from build123d import *

# Parameters (mm, degrees)
BOSS_EXTRUDE1_DEPTH     = 212
BOSS_EXTRUDE2_DEPTH     = 10
BOSS_EXTRUDE3_DEPTH     = 10
SKETCH4_R               = 3
CUT_EXTRUDE1_DEPTH      = 91
SKETCH6_R               = 7.5
CUT_EXTRUDE2_DEPTH      = 81
SKETCH7_R               = 1.5
SKETCH7_R_2             = 12.5
SKETCH7_W               = 10
SKETCH7_H               = 120
SKETCH7_W_2             = 60
SKETCH7_H_2             = 15
CUT_EXTRUDE3_DEPTH      = 12.5
CUT_EXTRUDE4_REACH      = 112.512
SKETCH8_R               = 12.5
SKETCH9_R               = 3
CUT_EXTRUDE5_DEPTH      = 26
CUT_EXTRUDE5_DEPTH_BACK = 66
SKETCH10_W              = 40
SKETCH10_H              = 6.35
CUT_EXTRUDE6_DEPTH      = 1
CUT_EXTRUDE6_DEPTH_BACK = 213
FILLET1_R               = 10


with BuildPart() as part:
    # Sketch1 → Boss-Extrude1 (new body)
    with BuildSketch(Plane.XY):
        Polygon((0, 0), (-20, 0), (-20, 20), (-242.984559153, 20), (-242.984559153, 25), (-260, 25), (-260, 30), (-49.158083864, 30), (-122.301669645, 77.5), (-242.984559153, 85), (-260, 85), (-260, 90), (-242.984559153, 90), (-110.511971445, 81.767313396), (0, 10), align=None)
    extrude(amount=BOSS_EXTRUDE1_DEPTH)

    # Sketch2 → Boss-Extrude2 (add)
    with BuildSketch(Plane(origin=(0, 0, 0), x_dir=(-1, 0, 0), z_dir=(0, 0, -1))):
        Polygon((0, 0), (260, 0), (260, 90), (110.511971445, 81.767313396), (0, 10), align=None)
    extrude(amount=-BOSS_EXTRUDE2_DEPTH)

    # Sketch3 → Boss-Extrude3 (add)
    with BuildSketch(Plane.XY.offset(212)):
        Polygon((-110.511971445, 81.767313396), (0, 10), (0, 0), (-260, 0), (-260, 90), align=None)
    extrude(amount=-BOSS_EXTRUDE3_DEPTH)

    # Sketch4 → Cut-Extrude1 (cut, through all)
    with BuildSketch(Plane.XZ):
        with Locations((-10, 187)):
            Circle(SKETCH4_R)
        with Locations((-10, 25)):
            Circle(SKETCH4_R)
    extrude(amount=-CUT_EXTRUDE1_DEPTH, mode=Mode.SUBTRACT)

    # Sketch6 → Cut-Extrude2 (cut, through all)
    with BuildSketch(Plane(origin=(0, 10, 0), x_dir=(-1, 0, 0), z_dir=(0, -1, 0))):
        with Locations((10, -25)):
            Circle(SKETCH6_R)
        with Locations((10, -187)):
            Circle(SKETCH6_R)
    extrude(amount=-CUT_EXTRUDE2_DEPTH, mode=Mode.SUBTRACT)

    # Sketch7 → Cut-Extrude3 (cut)
    with BuildSketch(Plane.XZ.offset(-20)):
        with Locations((-161.484559153, 161)):
            Circle(SKETCH7_R)
        with Locations((-225.684559153, 161)):
            Circle(SKETCH7_R)
        with Locations((-161.484559153, 51)):
            Circle(SKETCH7_R)
        with Locations((-225.684559153, 51)):
            Circle(SKETCH7_R)
        with Locations((-67.984559153, 136)):
            Circle(SKETCH7_R_2)
        with Locations((-92.099111311, 106)):
            Rectangle(SKETCH7_W, SKETCH7_H)
        with Locations((-70, 22.5)):
            Rectangle(SKETCH7_W_2, SKETCH7_H_2)
    extrude(amount=-CUT_EXTRUDE3_DEPTH, mode=Mode.SUBTRACT)

    # Sketch8 → Cut-Extrude4 (cut, up to next)
    with BuildSketch(Plane.ZY.offset(110.511971445), mode=Mode.PRIVATE) as cut_extrude4_sk1:
        with Locations((54, 57.25)):
            Circle(SKETCH8_R)
    cut_extrude4_tool1 = extrude(cut_extrude4_sk1.sketch, amount=-CUT_EXTRUDE4_REACH, mode=Mode.PRIVATE) & part.part
    add(cut_extrude4_tool1.solids().sort_by_distance((-110.511971, 57.25, 54))[0], mode=Mode.SUBTRACT)

    # Sketch9 → Cut-Extrude5 (cut, two sides)
    with BuildSketch(Plane.XZ.offset(-25)) as cut_extrude5_sk:
        with Locations((-251.5, 182)):
            Circle(SKETCH9_R)
        with Locations((-251.5, 30)):
            Circle(SKETCH9_R)
    extrude(amount=CUT_EXTRUDE5_DEPTH, mode=Mode.SUBTRACT)
    extrude(cut_extrude5_sk.sketch, amount=-CUT_EXTRUDE5_DEPTH_BACK, mode=Mode.SUBTRACT)

    # Sketch10 → Cut-Extrude6 (cut, two sides)
    with BuildSketch(Plane.XY.offset(212)) as cut_extrude6_sk:
        with Locations((-107.5, 3.175)):
            Rectangle(SKETCH10_W, SKETCH10_H)
    extrude(amount=CUT_EXTRUDE6_DEPTH, mode=Mode.SUBTRACT)
    extrude(cut_extrude6_sk.sketch, amount=-CUT_EXTRUDE6_DEPTH_BACK, mode=Mode.SUBTRACT)

    # Fillet1
    fillet1_edges = [part.edges().sort_by_distance(p)[0] for p in [
        (-110.511971445, 81.767313396, 106),
    ]]
    fillet(fillet1_edges, radius=FILLET1_R)


solid = part.part
Design review of the part built by this model. Coordinates are the model's own, in mm. A direction names the side the tool comes from. Round coordinates to 2 decimals unless told otherwise and drop trailing zeros. Loops run counter-clockwise (first coordinate to the right, second up) from the corner with the lowest first, then second, coordinate; pieces in that order, holes last. Notation, with made-up numbers: (38, 20.5) -> (68, 20.5) arc R27 ccw to (68, 44.5) -> close; hole circle Ø2 at (11, 50). An arc over 180 degrees is marked (long way). Use one line per item in the form item = value. Start each with the question number.
Q1. For pin 1 Ø6 at (x, z) = (-161, 100.5) entering from +Y; pin 2 Ø1.5 at (x, z) = (-110.5, 59.5) entering from +Y; pin 3 Ø2 at (y, z) = (74.5, 108.5) entering from +X; pin 4 Ø5.5 at (x, z) = (-251.5, 182) entering from -Y, all flat-tipped, find the tip position at first contact; note any pin that passes through.
Q2. We need section C-C on y = 65.5. Give the boundary of the cut face in (x, z), then the cut area to 3 significant figures.
Q3. We need section B-B on z = 117. Give the boundary of the cut face in (x, y), then the cut area to 3 significant figures.
Q4. We need section A-A on x = -251.5. Give the boundary of the cut face in (y, z), then the cut area to 3 significant figures.
Q5. Draft analysis for pull direction X (two halves, no side actions). For faces 6 (the face through (-157, 36, 212)), 7 (the face through (-108, 6.35, 5)), 8 (the face through (-20, 10, 105)), state which applies: +X half, -X half, draft (parallel to the pull), parting line (faces both ways), or undercut.
Q6. Wall thickness on line 1 along Z through (x, y) = (-251, 28); line 2 along Z through (x, y) = (-207, 10); line 3 along Y through (x, z) = (-190.5, 166.5): over which ranges is each line inside the solid? List them lowest first. Write a range as [from, to].
Q7. Machinability: for faces 1 (the face through (-17.154, 14.34, 22.747)), 2 (the face through (-127.5, 3, 207)), 3 (the face through (-87.099, 25, 105)), 4 (the face through (0, 5, 105)), 5 (the face through (-47, 32.5, 23)), which of the approach directions +Z, -Z, +X, -X, +Y, -Y give a long, thin tool a straight path to every point of the face, cutting with its end or side? Answer none if there is none.
Q8. We need section D-D on x = -10. Give the boundary of the cut face in (y, z).
Calculated:
q1.pin_1 = 85.09
q1.pin_2 = 81.63
q1.pin_3 = -97.78
q1.pin_4 = through
q2.outline = (-260, 0) -> (-85.46, 0) -> (-85.46, 44.61) -> (-103.82, 44.61) -> (-103.82, 10) -> (-260, 10) -> close; (-260, 202) -> (-103.82, 202) -> (-103.82, 63.39) -> (-85.46, 63.39) -> (-85.46, 212) -> (-260, 212) -> close
q2.area = 6,670 mm²
q3.outline = (-260, 25) -> (-242.98, 25) -> (-242.98, 20) -> (-97.1, 20) -> (-97.1, 30) -> (-260, 30) -> close; (-260, 85) -> (-242.98, 85) -> (-122.3, 77.5) -> (-49.16, 30) -> (-87.1, 30) -> (-87.1, 20) -> (-20, 20) -> (-20, 0) -> (0, 0) -> (0, 10) -> (-108.31, 80.34) arc R10 ccw to (-113.13, 81.93) -> (-242.98, 90) -> (-260, 90) -> close
q3.area = 4,140 mm²
q4.outline = (0, 0) -> (90, 0) -> (90, 27) -> (85, 27) -> (85, 10) -> (30, 10) -> (30, 27) -> (25, 27) -> (25, 10) -> (0, 10) -> close; (0, 202) -> (25, 202) -> (25, 185) -> (30, 185) -> (30, 202) -> (85, 202) -> (85, 185) -> (90, 185) -> (90, 212) -> (0, 212) -> close; (25, 33) -> (30, 33) -> (30, 179) -> (25, 179) -> close; (85, 33) -> (90, 33) -> (90, 179) -> (85, 179) -> close
q4.area = 3,600 mm²
q5.face_6 = draft
q5.face_7 = undercut
q5.face_8 = -X half
q6.line_1 = [0, 27.04], [32.96, 179.04], [184.96, 212]
q6.line_2 = [0, 10], [202, 212]
q6.line_3 = [20, 30], [81.74, 86.74]
q7.face_1 = +Y
q7.face_2 = +Z, -Z, -Y
q7.face_3 = -Y
q7.face_4 = +Z, -Z, +X, +Y, -Y
q7.face_5 = -X, -Y
q8.outline = (0, 0) -> (16.49, 0) -> (16.49, 17.5) -> (10, 17.5) -> (10, 22) -> (0, 22) -> close; (0, 28) -> (10, 28) -> (10, 32.5) -> (16.49, 32.5) -> (16.49, 179.5) -> (10, 179.5) -> (10, 184) -> (0, 184) -> close; (0, 190) -> (10, 190) -> (10, 194.5) -> (16.49, 194.5) -> (16.49, 212) -> (0, 212) -> close
